from build123d import *

# Parameters (mm, degrees)
ESQUISSE1_W                                    = 26
ESQUISSE1_H                                    = 27.3
BOSS_EXTRU_1_DEPTH                             = 2.1
ESQUISSE2_R                                    = 11.8
BOSS_EXTRU_2_DEPTH                             = 40
ESQUISSE3_W                                    = 26
ESQUISSE3_H                                    = 2.1
BOSS_EXTRU_3_DEPTH                             = 3.7
ESQUISSE4_R                                    = 11.8
BOSS_EXTRU_4_DEPTH                             = 2.8
D_GAGEMENT_M181_D                              = 20.9
D_GAGEMENT_M181_DEPTH                          = 13.9
ESQUISSE7_R                                    = 8.75
BOSS_EXTRU_5_DEPTH                             = 10.7
ENL_V_MAT_EXTRU_1_DEPTH                        = 10.8
ESQUISSE9_W                                    = 5.1
ESQUISSE9_H                                    = 1.25
ENL_V_MAT_EXTRU_2_DEPTH                        = 0.5
ENL_V_MAT_EXTRU_3_DEPTH                        = 30.9
BOSS_EXTRU_6_DEPTH                             = 30.9
ENL_V_MAT_EXTRU_4_DEPTH                        = 30.9
BOSS_EXTRU_7_DEPTH                             = 30.9
BOSS_EXTRU_8_DEPTH                             = 30.9
BOSS_EXTRU_9_DEPTH                             = 30.9
ENL_V_MAT_EXTRU_5_REACH                        = 16.1
ENL_V_MAT_EXTRU_6_REACH                        = 16.1
ESQUISSE20_W                                   = 5.5
ESQUISSE20_H                                   = 9.8
ENL_V_MAT_EXTRU_7_DEPTH                        = 25.725
BOSS_EXTRU_10_REACH                            = 31.279
ESQUISSE21_W                                   = 1.4
ESQUISSE21_H                                   = 4.4
FRAISAGE_POUR_VIS_T_TE_FRAIS_E_M31_D           = 3.5
FRAISAGE_POUR_VIS_T_TE_FRAIS_E_M31_DEPTH       = 42.1
FRAISAGE_POUR_VIS_T_TE_FRAIS_E_M31_CSINK_D     = 6.099893765
FRAISAGE_POUR_VIS_T_TE_FRAIS_E_M31_CSINK_ANGLE = 89.999002
CONG_1_R                                       = 3.5


with BuildPart() as part:
    # Esquisse1 → Boss.-Extru.1 (new body)
    with BuildSketch(Plane(origin=(0, 0, 0), x_dir=(-1, 0, 0), z_dir=(0, 0, -1))):
        with Locations((0, -1.85)):
            Rectangle(ESQUISSE1_W, ESQUISSE1_H)
    extrude(amount=-BOSS_EXTRU_1_DEPTH)

    # Esquisse2 → Boss.-Extru.2 (add)
    with BuildSketch(Plane.XY.offset(2.1)):
        Circle(ESQUISSE2_R)
    extrude(amount=BOSS_EXTRU_2_DEPTH)

    # Esquisse3 → Boss.-Extru.3 (add)
    with BuildSketch(Plane(origin=(0, 11.8, 0), x_dir=(-1, 0, 0), z_dir=(0, 1, 0))):
        with Locations((0, 1.05)):
            Rectangle(ESQUISSE3_W, ESQUISSE3_H)
    extrude(amount=BOSS_EXTRU_3_DEPTH)

    # Esquisse4 → Boss.-Extru.4 (add)
    with BuildSketch(Plane(origin=(0, 0, 0), x_dir=(-1, 0, 0), z_dir=(0, 0, -1))):
        Circle(ESQUISSE4_R)
    extrude(amount=BOSS_EXTRU_4_DEPTH)

    # Dégagement M181
    with Locations(Plane(origin=(0, 0, -2.8), x_dir=(-1, 0, 0), z_dir=(0, 0, -1))):
        with Locations((0, 0)):
            Hole(D_GAGEMENT_M181_D / 2, depth=D_GAGEMENT_M181_DEPTH)

    # Esquisse7 → Boss.-Extru.5 (add)
    with BuildSketch(Plane(origin=(0, 0, 11.1), x_dir=(-1, 0, 0), z_dir=(0, 0, -1))):
        Circle(ESQUISSE7_R)
    extrude(amount=BOSS_EXTRU_5_DEPTH)

    # Esquisse8 → Enlèv. mat.-Extru.1 (cut)
    with BuildSketch(Plane(origin=(0, 0, 0.4), x_dir=(-1, 0, 0), z_dir=(0, 0, -1))):
        Polygon((6.35, -3.8), (6.35, 3.8), (-6.35, 3.8), (-6.35, -3.8), (-3.65, -3.8), (-3.65, -5.6), (-2.55, -5.6), (-2.55, -6.9), (2.55, -6.9), (2.55, -5.6), (3.65, -5.6), (3.65, -3.8), align=None)
    extrude(amount=-ENL_V_MAT_EXTRU_1_DEPTH, mode=Mode.SUBTRACT)

    # Esquisse9 → Enlèv. mat.-Extru.2 (cut)
    with BuildSketch(Plane(origin=(0, 0, 11.2), x_dir=(-1, 0, 0), z_dir=(0, 0, -1))):
        with Locations((0, -6.275)):
            Rectangle(ESQUISSE9_W, ESQUISSE9_H)
    extrude(amount=-ENL_V_MAT_EXTRU_2_DEPTH, mode=Mode.SUBTRACT)

    # Esquisse10 → Enlèv. mat.-Extru.3 (cut)
    with BuildSketch(Plane.XY.offset(42.1)):
        with BuildLine():
            Line((-11.725, -1.328297783), (-11.725, 1.328297783))
            ThreePointArc((-11.725, 1.328297783), (-11.8, 0), (-11.725, -1.328297783))
        make_face()
    extrude(amount=-ENL_V_MAT_EXTRU_3_DEPTH, mode=Mode.SUBTRACT)

    # Esquisse11 → Boss.-Extru.6 (add)
    with BuildSketch(Plane.XY.offset(42.1)):
        with BuildLine():
            Line((-9.536115561, 6.95), (-11.725, 6.95))
            Line((-11.725, 6.95), (-11.725, 1.328297783))
            ThreePointArc((-11.725, 1.328297783), (-10.995892082, 4.281396655), (-9.536115561, 6.95))
        make_face()
    extrude(amount=-BOSS_EXTRU_6_DEPTH)

    # Esquisse12 → Enlèv. mat.-Extru.4 (cut)
    with BuildSketch(Plane.XY.offset(42.1)):
        with BuildLine():
            Line((11.725, 1.328297783), (11.725, -1.328297783))
            ThreePointArc((11.725, -1.328297783), (11.8, 0), (11.725, 1.328297783))
        make_face()
    extrude(amount=-ENL_V_MAT_EXTRU_4_DEPTH, mode=Mode.SUBTRACT)

    # Esquisse13 → Boss.-Extru.7 (add)
    with BuildSketch(Plane.XY.offset(42.1)):
        with BuildLine():
            Line((11.725, 1.328297783), (11.725, 6.95))
            Line((11.725, 6.95), (9.536115561, 6.95))
            ThreePointArc((9.536115561, 6.95), (10.995892082, 4.281396655), (11.725, 1.328297783))
        make_face()
    extrude(amount=-BOSS_EXTRU_7_DEPTH)

    # Esquisse14 → Boss.-Extru.8 (add)
    with BuildSketch(Plane.XY.offset(42.1)):
        with BuildLine():
            Line((-11.725, -1.328297783), (-11.725, -5.65))
            Line((-11.725, -5.65), (-10.359416007, -5.65))
            ThreePointArc((-10.359416007, -5.65), (-11.251650328, -3.555329084), (-11.725, -1.328297783))
        make_face()
    extrude(amount=-BOSS_EXTRU_8_DEPTH)

    # Esquisse15 → Boss.-Extru.9 (add)
    with BuildSketch(Plane.XY.offset(42.1)):
        with BuildLine():
            Line((10.359416007, -5.65), (11.725, -5.65))
            Line((11.725, -5.65), (11.725, -1.328297783))
            ThreePointArc((11.725, -1.328297783), (11.251650328, -3.555329084), (10.359416007, -5.65))
        make_face()
    extrude(amount=-BOSS_EXTRU_9_DEPTH)

    # Esquisse17 → Enlèv. mat.-Extru.5 (cut, up to next)
    with BuildSketch(Plane(origin=(0, 0, 28), x_dir=(-1, 0, 0), z_dir=(0, 0, -1)), mode=Mode.PRIVATE) as enl_v_mat_extru_5_sk1:
        with BuildLine():
            Line((-9.536115561, 6.95), (9.536115561, 6.95))
            ThreePointArc((9.536115561, 6.95), (0, 11.8), (-9.536115561, 6.95))
        make_face()
    enl_v_mat_extru_5_tool1 = extrude(enl_v_mat_extru_5_sk1.sketch, amount=-ENL_V_MAT_EXTRU_5_REACH, mode=Mode.PRIVATE) & part.part
    add(enl_v_mat_extru_5_tool1.solids().sort_by_distance((0, 8.928831, 28))[0], mode=Mode.SUBTRACT)

    # Esquisse19 → Enlèv. mat.-Extru.6 (cut, up to next)
    with BuildSketch(Plane(origin=(0, 0, 28), x_dir=(-1, 0, 0), z_dir=(0, 0, -1)), mode=Mode.PRIVATE) as enl_v_mat_extru_6_sk1:
        with BuildLine():
            Line((10.359416007, -5.65), (-10.359416007, -5.65))
            ThreePointArc((-10.359416007, -5.65), (0, -11.8), (10.359416007, -5.65))
        make_face()
    enl_v_mat_extru_6_tool1 = extrude(enl_v_mat_extru_6_sk1.sketch, amount=-ENL_V_MAT_EXTRU_6_REACH, mode=Mode.PRIVATE) & part.part
    add(enl_v_mat_extru_6_tool1.solids().sort_by_distance((0, -8.174843, 28))[0], mode=Mode.SUBTRACT)

    # Esquisse20 → Enlèv. mat.-Extru.7 (cut, through all)
    with BuildSketch(Plane.ZY.offset(11.725)):
        with Locations((39.35, 2.05)):
            Rectangle(ESQUISSE20_W, ESQUISSE20_H)
    extrude(amount=-ENL_V_MAT_EXTRU_7_DEPTH, mode=Mode.SUBTRACT)

    # Esquisse21 → Boss.-Extru.10 (add, up to next)
    with BuildSketch(Plane.XZ.offset(13.779218989), mode=Mode.PRIVATE) as boss_extru_10_sk1:
        with Locations((0, 25.8)):
            Rectangle(ESQUISSE21_W, ESQUISSE21_H)
    boss_extru_10_tool1 = extrude(boss_extru_10_sk1.sketch, amount=-BOSS_EXTRU_10_REACH, mode=Mode.PRIVATE) - part.part
    add(boss_extru_10_tool1.solids().sort_by_distance((0, -13.779219, 25.8))[0])

    # Fraisage pour vis à tête fraisée M31
    with Locations(Plane(origin=(0, 0, 0), x_dir=(-1, 0, 0), z_dir=(0, 0, -1))):
        with Locations((-9.5, 12), (9.5, -12)):
            CounterSinkHole(FRAISAGE_POUR_VIS_T_TE_FRAIS_E_M31_D / 2, FRAISAGE_POUR_VIS_T_TE_FRAIS_E_M31_CSINK_D / 2, depth=FRAISAGE_POUR_VIS_T_TE_FRAIS_E_M31_DEPTH, counter_sink_angle=FRAISAGE_POUR_VIS_T_TE_FRAIS_E_M31_CSINK_ANGLE)

    # Congé1
    cong_1_edges = [part.edges().sort_by_distance(p)[0] for p in [
        (13, 15.5, 1.05),
        (-13, 15.5, 1.05),
        (-13, -15.5, 1.05),
        (13, -15.5, 1.05),
    ]]
    fillet(cong_1_edges, radius=CONG_1_R)


solid = part.part
Geometry: final body of the model. Coordinates: model frame, mm. A direction names the side the tool comes from. Round coordinates to 2 decimals unless told otherwise and drop trailing zeros. Order: outer loops, then holes, each group sorted by start corner. A loop starts at its lowest first (then second) coordinate and runs counter-clockwise, first axis right, second up. Notation, with made-up numbers: (-8, 60) - (21, 60) arc R18 ccw to (21, 95) - close; hole circle Ø11 at (-21.75, 58.5). An arc over 180 degrees is marked (long way). Write each question's results on one line, items separated by ' | '.
Item 1: Reachability of faces 4 (the flat face through (0, 9, 28)), 5 (the flat face through (-11.4, -4.4, 11.2)), 6 (the flat face through (5, -8, 11.1)), 7 (the flat face through (-11, 5, 11.2)) from +Z, -Z, +X, -X, +Y, -Y: full face, straight path, thin tool, end or side. Return the list, or none.
Completed:
face 4: +Z, +X, -X, +Y | face 5: -X, -Y | face 6: -Z | face 7: -X, +Y
Item 2: First-contact query: pin 1 Ø12 at (x, z) = (9.5, 34.5) entering from -Y; pin 2 Ø1.4 at (y, z) = (-6.5, 5.5) entering from +X; pin 3 Ø4 at (y, z) = (-6, 17) entering from +X (3 decimals). Flat tips, straight axial feed; report the tip coordinate or a pass-through.
Completed:
pin 1: y = -5.65 | pin 2: x = 10.28 | pin 3: x = 11.725
Item 3: Section C-C, the plane z = 16.5. Return the cut outline in (x, y) (3 decimals).
Completed:
outline: (-11.725, -5.65) - (-10.359, -5.65) arc R11.8 ccw to (10.359, -5.65) - (11.725, -5.65) - (11.725, 6.95) - (9.536, 6.95) arc R11.8 ccw to (-9.536, 6.95) - (-11.725, 6.95) - close
Item 4: Mould query, pull axis Y, two halves, no side actions, for faces 1 (the flat face through (0, -6.9, 6)), 2 (the flat face through (0, -5.65, 34)), 3 (the flat face through (11, 5, 11.2)). Classes: pulls with the +Y half, pulls with the -Y half, needs draft (parallel to the pull), parting line crosses it, or undercut.
Completed:
face 1: undercut | face 2: pulls with the -Y half | face 3: needs draft
Item 5: Section A-A, the plane z = 7.5. Return the cut outline in (x, y), and give its area (3 significant figures).
Completed:
outline: circle Ø23.6 at (0, 0); circle Ø17.5 at (0, 0); hole circle Ø20.9 at (0, 0); hole (-6.35, -3.8) - (-3.65, -3.8) - (-3.65, -5.6) - (-2.55, -5.6) - (-2.55, -6.9) - (2.55, -6.9) - (2.55, -5.6) - (3.65, -5.6) - (3.65, -3.8) - (6.35, -3.8) - (6.35, 3.8) - (-6.35, 3.8) - close | area: 219 mm^2
Item 6: Section D-D, the plane y = -2. Return the cut outline in (x, z) (3 decimals).
Completed:
outline: (-13, 0) - (-11.629, 0) - (-11.629, -2.8) - (-10.257, -2.8) - (-10.257, 11.1) - (-8.518, 11.1) - (-8.518, 0.4) - (-6.35, 0.4) - (-6.35, 11.2) - (6.35, 11.2) - (6.35, 0.4) - (8.518, 0.4) - (8.518, 11.1) - (10.257, 11.1) - (10.257, -2.8) - (11.629, -2.8) - (11.629, 0) - (13, 0) - (13, 2.1) - (11.629, 2.1) - (11.629, 11.2) - (11.725, 11.2) - (11.725, 36.6) - (-11.725, 36.6) - (-11.725, 11.2) - (-11.629, 11.2) - (-11.629, 2.1) - (-13, 2.1) - close
Item 7: Material intervals for line 1 along Y through (x, z) = (0, 2.5); line 2 along Y through (x, z) = (0, 1.25); line 3 along X through (y, z) = (-12, 1.7), sorted ascending. Write a range as [from, to].
Completed:
line 1: [-11.8, -10.45], [-8.75, -6.9], [3.8, 8.75], [10.45, 11.8] | line 2: [-15.5, -10.45], [-8.75, -6.9], [3.8, 8.75], [10.45, 15.5] | line 3: [-13, -11.25], [-7.75, 13]
